Read the model definition and answer for the solid it produces. Units are mm, in the model's axes. A direction names the side the tool comes from. Coordinates: 2 decimals unless noted, no trailing zeros. Write each loop counter-clockwise with the first axis right and the second up, starting at its lowest first coordinate (ties: lowest second). Pieces come first, ordered by that corner, then holes.
from build123d import *

# Parameters (mm, degrees)
RESSALTO_EXTRUS_O1_DEPTH = 1
ESBO_O3_R                = 0.225
RESSALTO_EXTRUS_O3_DEPTH = 29
ESBO_O4_R                = 0.225
RESSALTO_EXTRUS_O4_DEPTH = 24.775


# Read off the part's stored shape, not the designer's step: Ressalto-extrusão2
with BuildPart() as part:
    # Esboço1 → Ressalto-extrusão1 (new body)
    with BuildSketch(Plane.XZ):
        with BuildLine():
            Line((1.5, -1.116646766), (1.5, 1.116646766))
            ThreePointArc((1.5, 1.116646766), (-1.87, 0), (1.5, -1.116646766))
        make_face()
    extrude(amount=-RESSALTO_EXTRUS_O1_DEPTH)

    # Ressalto-extrusão2 outline → Ressalto-extrusão2 (revolve)
    with BuildSketch(Plane.XY):
        with BuildLine():
            Line((1.5, 1), (1.5, 3.99))
            ThreePointArc((1.5, 3.99), (1.060660172, 5.050660172), (0, 5.49))
            Line((0, 5.49), (0, 1))
            Line((0, 1), (1.5, 1))
        make_face()
    revolve(axis=Axis((0, 0, 0), (0, 1, 0)))

    # Esboço3 → Ressalto-extrusão3 (add)
    with BuildSketch(Plane.XZ):
        with Locations(Location((-1.27, 0, 0), (0, 0, 270))):
            Circle(ESBO_O3_R)
    extrude(amount=RESSALTO_EXTRUS_O3_DEPTH)

    # Esboço4 → Ressalto-extrusão4 (add)
    with BuildSketch(Plane.XZ):
        with Locations(Location((1.27, 0, 0), (0, 0, 270))):
            Circle(ESBO_O4_R)
    extrude(amount=RESSALTO_EXTRUS_O4_DEPTH)


solid = part.part
Item 1: Find the intervals of material crossed by probe 1 along X at (y, z) = (-4, 0) (3 decimals); probe 2 along Y at (x, z) = (-1.6, -0.1); probe 3 along Y at (x, z) = (0.15, 1.25), in increasing order.
Item 2: The part is cut by section D-D (y = 1.5). Give the vertices of the cut face in (x, z), and give its area (3 significant figures).
Item 3: The part is cut by section C-C (y = -26). Give the vertices of the cut face in (x, z) (3 decimals).
Item 4: Given pin 1 (1.5 mm diameter, centred on x = -1, z = -1, fed in from -Y); pin 2 (2 mm diameter, centred on y = -1, z = -0.5, fed in from +X) (3 decimals); pin 3 (1.5 mm diameter, centred on x = 0, y = -22.5, fed in from -Z), each flat-ended and moving along its own axis, determine where each tip first touches the part or whether it passes through.
Item 5: The part is cut by section B-B (y = -15.5). Give the vertices of the cut face in (x, z) (3 decimals).
Item 6: The part is cut by section A-A (x = 0). Give the vertices of the cut face in (y, z), and give its area (3 significant figures).
Item 7: For faces 1 (the cylindrical face through (-1.87, 0.49, 0.07)), 2 (the cylindrical face through (-1.5, 2.52, -0.07)), determine the directions among +Z, -Z, +X, -X, +Y, -Y from which every point of the face is accessible in a straight line to the end or side of a thin tool.
Answer:
1. probe 1: x = -1.495 to -1.045, 1.045 to 1.495
1. probe 2: y = 0 to 1
1. probe 3: y = 0 to 4.81
2. outline: circle Ø3 at (0, 0)
2. area: 7.07 mm2
3. outline: circle Ø0.45 at (-1.27, 0)
4. pin 1: stops at y = 0
4. pin 2: stops at x = 1.495
4. pin 3: passes through
5. outline: circle Ø0.45 at (-1.27, 0); circle Ø0.45 at (1.27, 0)
6. outline: (0, -1.87) - (1, -1.87) - (1, -1.5) - (3.99, -1.5) arc R1.5 ccw to (3.99, 1.5) - (1, 1.5) - (1, 1.87) - (0, 1.87) - close
6. area: 16.2 mm2
7. face 1: +Y, -Y
7. face 2: +Y
